```python
from build123d import *

# Parameters (mm, degrees)
SKETCH1_W           = 60
SKETCH1_H           = 120
BOSS_EXTRUDE1_DEPTH = 4
SKETCH2_R           = 4
CUT_EXTRUDE1_DEPTH  = 4
SKETCH3_R           = 25
BOSS_EXTRUDE2_DEPTH = 25
SKETCH4_R           = 21.6
CUT_EXTRUDE2_DEPTH  = 25
SKETCH5_R           = 11
CUT_EXTRUDE3_DEPTH  = 25


with BuildPart() as part:
    # Sketch1 → Boss-Extrude1 (new body)
    with BuildSketch(Plane.XY):
        Rectangle(SKETCH1_W, SKETCH1_H)
    extrude(amount=BOSS_EXTRUDE1_DEPTH)

    # Sketch2 → Cut-Extrude1 (cut)
    with BuildSketch(Plane.XY.offset(4)):
        with Locations((-20, 50)):
            Circle(SKETCH2_R)
        with Locations((20, 50)):
            Circle(SKETCH2_R)
        with Locations((20, -50)):
            Circle(SKETCH2_R)
        with Locations((-20, -50)):
            Circle(SKETCH2_R)
    extrude(amount=-CUT_EXTRUDE1_DEPTH, mode=Mode.SUBTRACT)

    # Sketch3 → Boss-Extrude2 (add)
    with BuildSketch(Plane.XY.offset(4)):
        Circle(SKETCH3_R)
    extrude(amount=BOSS_EXTRUDE2_DEPTH)

    # Sketch4 → Cut-Extrude2 (cut)
    with BuildSketch(Plane(origin=(0, 0, 0), x_dir=(-1, 0, 0), z_dir=(0, 0, -1))):
        Circle(SKETCH4_R)
    extrude(amount=-CUT_EXTRUDE2_DEPTH, mode=Mode.SUBTRACT)

    # Sketch5 → Cut-Extrude3 (cut)
    with BuildSketch(Plane.XY.offset(29)):
        Circle(SKETCH5_R)
    extrude(amount=-CUT_EXTRUDE3_DEPTH, mode=Mode.SUBTRACT)


solid = part.part
```
The model under review builds one solid part; all positions refer to its coordinate system, in mm. A direction names the side the tool comes from. Round coordinates to 2 decimals unless told otherwise and drop trailing zeros. Order: outer loops, then holes, each group sorted by start corner. A loop starts at its lowest first (then second) coordinate and runs counter-clockwise, first axis right, second up.
(1) Wall thickness on L1, parallel to Y at x = 0, z = 18.5; L2, parallel to Z at x = 4.5, y = -55; L3, parallel to Y at x = 7, z = 16.5: over which ranges is each line inside the solid? List them lowest first.
Working result:
L1: y = -25 to -21.6, 21.6 to 25
L2: z = 0 to 4
L3: y = -24 to -20.43, 20.43 to 24
(2) Take a section at C-C, the plane y = 0. State the section outline as (x, z) points.
Working result:
outline: (-30, 0) - (-21.6, 0) - (-21.6, 25) - (-11, 25) - (-11, 29) - (-25, 29) - (-25, 4) - (-30, 4) - close; (11, 25) - (21.6, 25) - (21.6, 0) - (30, 0) - (30, 4) - (25, 4) - (25, 29) - (11, 29) - close
(3) Take a section at B-B, the plane x = 0. State the section outline as (y, z) points, plus the area to 3 significant figures.
Working result:
outline: (-60, 0) - (-21.6, 0) - (-21.6, 25) - (-11, 25) - (-11, 29) - (-25, 29) - (-25, 4) - (-60, 4) - close; (11, 25) - (21.6, 25) - (21.6, 0) - (60, 0) - (60, 4) - (25, 4) - (25, 29) - (11, 29) - close
area: 562 mm2
(4) For P1, Ø1, axis at x = 16.5, y = -36, coming from the +Z side; P2, Ø7, axis at x = -20, y = -50, coming from the +Z side; P3, Ø6, axis at x = 19, z = 15, coming from the +Y side; P4, Ø1, axis at x = -15.5, z = 24.5, coming from the -Y side, all flat-tipped, find the tip position at first contact; note any pin that passes through.
Working result:
P1: stops at z = 4
P2: passes through
P3: stops at y = 19.21
P4: stops at y = -20
(5) Mouldability with a two-part tool opening along X and no side actions: class faces 4 (the face through (0, 60, 2)), 5 (the face through (-30, -1, 2)), 6 (the face through (-2.38, -10.74, 27.03)) as released by +X, released by -X, zero draft, split by the parting line, or undercut.
Working result:
face 4: zero draft
face 5: released by -X
face 6: undercut
(6) Take a section at D-D, the plane x = 19. State the section outline as (y, z) points.
Working result:
outline: (-60, 0) - (-53.87, 0) - (-53.87, 4) - (-60, 4) - close; (-46.13, 0) - (-10.27, 0) - (-10.27, 25) - (10.27, 25) - (10.27, 0) - (46.13, 0) - (46.13, 4) - (16.25, 4) - (16.25, 29) - (-16.25, 29) - (-16.25, 4) - (-46.13, 4) - close; (53.87, 0) - (60, 0) - (60, 4) - (53.87, 4) - close
(7) Take a section at A-A, the plane y = -50. State the section outline as (x, z) points, plus the area to 3 significant figures.
Working result:
outline: (-30, 0) - (-24, 0) - (-24, 4) - (-30, 4) - close; (-16, 0) - (16, 0) - (16, 4) - (-16, 4) - close; (24, 0) - (30, 0) - (30, 4) - (24, 4) - close
area: 176 mm2
(8) Tool access review of faces 1 (the face through (30, -1, 2)), 2 (the face through (23.846, 7.509, 16.325)), 3 (the face through (10, 5, 25)): name each direction out of +Z, -Z, +X, -X, +Y, -Y from which nothing blocks a thin tool from reaching the whole face with its end or side.
Working result:
face 1: +Z, -Z, +X, +Y, -Y
face 2: +Z
face 3: -Z
